```python
from build123d import *

# Parameters (mm, degrees)
F0_W      = 36
F0_H      = 2
F1_DEPTH  = 2
F0_W_2    = 4.0826744884
F0_H_2    = 5.745283328
F2_DEPTH  = 8.5
F3_DEPTH  = 11
F0_W_3    = 2
F4_DEPTH  = 11
F5_W      = 3
F5_H      = 5.745283328
F5_W_2    = 2
F5_W_3    = 1
F6_DEPTH  = 2
F8_DEPTH  = 5.745283328
F10_DEPTH = 5.745283328
F0_W_4    = 3.3082471341
F11_DEPTH = 8


# Not quite as in the source:
# - a feature names something its author has since deleted; it is built from what else it names


with BuildPart() as f1:
    # F0 (on Top) → F1 (new body)
    with BuildSketch(Plane.XY):
        with Locations((0, -10)):
            Rectangle(F0_W, F0_H)
        Polygon((-18, -9), (18, -9), (18, -2.872641664), (14.6917528659, -2.872641664), (14.6917528659, 2.872641664), (18, 2.872641664), (18, 9), (-18, 9), (-18, 2.872641664), (-13.9173255116, 2.872641664), (-13.9173255116, -2.872641664), (-18, -2.872641664), align=None)
    extrude(amount=F1_DEPTH)

    # F0 (on Top) → F2 (join)
    with BuildSketch(Plane.XY):
        with Locations((-15.9586627558, 0)):
            Rectangle(F0_W_2, F0_H_2)
    extrude(amount=F2_DEPTH)

    # F0 (on Top) → F3 (join)
    with BuildSketch(Plane.XY):
        with Locations((0, -10)):
            Rectangle(F0_W, F0_H)
        with Locations((0, 10)):
            Rectangle(F0_W, F0_H)
    extrude(amount=F3_DEPTH)

    # F0 (on Top) → F4 (join)
    with BuildSketch(Plane.XY):
        with Locations((-19, 0)):
            Rectangle(F0_W_3, F0_H_2)
        with Locations((19, 0)):
            Rectangle(F0_W_3, F0_H_2)
    extrude(amount=F4_DEPTH)

    # F5 (on face) → F6 (join)
    with BuildSketch(Plane.XY.offset(11)):
        with Locations((18.5, 0)):
            Rectangle(F5_W, F5_H)
        with Locations((-19, 0)):
            Rectangle(F5_W_2, F5_H)
        with Locations((-17.5, 0)):
            Rectangle(F5_W_3, F5_H)
    extrude(amount=F6_DEPTH)

    # F7 (on face) → F8 (cut, through all)
    with BuildSketch(Plane.XZ.offset(2.872641664)):
        Polygon((-20, 13), (-17, 11), (-17, 13), align=None)
    extrude(amount=-F8_DEPTH, mode=Mode.SUBTRACT)

    # F9 (on face) → F10 (cut, through all)
    with BuildSketch(Plane.XZ.offset(2.872641664)):
        Polygon((17, 13), (17, 11), (20, 13), align=None)
    extrude(amount=-F10_DEPTH, mode=Mode.SUBTRACT)

    # F0 (on Top) → F11 (join)
    with BuildSketch(Plane.XY):
        with Locations((16.345876433, 0)):
            Rectangle(F0_W_4, F0_H_2)
    extrude(amount=F11_DEPTH)


solid = f1.part
```
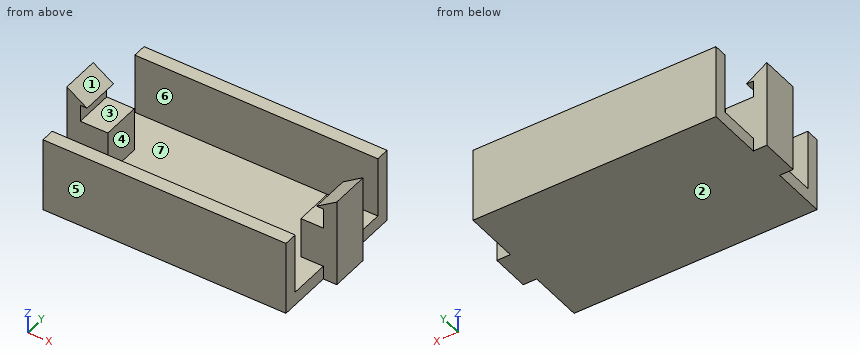
Design review of the part built by this model. Coordinates are the model's own, in mm. Face numbers are marked on the shaded views. A direction names the side the tool comes from. Give positions to 0.01 mm unless a question says otherwise; leave off trailing zeros. Loops run counter-clockwise (first coordinate to the right, second up) from the corner with the lowest first, then second, coordinate; pieces in that order, holes last. Notation, with made-up numbers: M 46.25,6 L 82.25,6 A29 cw 82.25,28 Z; hole C 8.25,9 d6. An arc over 180 degrees is marked long. Return JSON: item names as keys, results as strings. Group by question number.
Item 1: Tool access review of the marked faces 5, 6 and 7: name each direction out of +Z, -Z, +X, -X, +Y, -Y from which nothing blocks a thin tool from reaching the whole face with its end or side.
Item 2: Mouldability with a two-part tool opening along Z and no side actions: class the marked faces 1, 2, 3 and 4 as released by +Z, released by -Z, zero draft, split by the parting line, or undercut.
Item 3: Insertion check: pin 1 Ø3.5 at (x, y) = (-16, -0.5) entering from +Z; pin 2 Ø6.5 at (y, z) = (7, 7) entering from -X; pin 3 Ø1 at (x, y) = (15.5, -1) entering from +Z. Each pin has a flat end and moves straight along its axis. Give the tip position at first contact, or say it passes through.
Item 4: For probe 1 along Y at (x, z) = (-16.5, 4); probe 2 along X at (y, z) = (2.5, 6); probe 3 along Y at (x, z) = (-9.5, 9), list the stretches that pass through material, from the lowest coordinate up.
Item 5: We need section A-A (z = 4.75). Give the boundary of the cut face in (x, y).
Item 6: We need section D-D (z = 1.25). Give the boundary of the cut face in (x, y).
Item 7: We need section C-C (x = 5). Give the boundary of the cut face in (y, z), and give its area (3 significant figures).
Item 8: We need section B-B (y = 1.5). Give the boundary of the cut face in (x, z).
Output:
{
 "1": {"face 5": "+Z, -Z, +X, -X, -Y", "face 6": "+Z, +X, -X", "face 7": "+Z"},
 "2": {"face 1": "released by +Z", "face 2": "released by -Z", "face 3": "undercut", "face 4": "zero draft"},
 "3": {"pin 1": "stops at z = 11.5", "pin 2": "stops at x = -18", "pin 3": "stops at z = 8"},
 "4": {"probe 1": "y = -11 to -9, -2.87 to 2.87, 9 to 11", "probe 2": "x = -20 to -13.92, 14.69 to 20", "probe 3": "y = -11 to -9, 9 to 11"},
 "5": {"outline": "M -20,-2.87 L -13.92,-2.87 L -13.92,2.87 L -20,2.87 Z; M -18,-11 L 18,-11 L 18,-9 L -18,-9 Z; M -18,9 L 18,9 L 18,11 L -18,11 Z; M 14.69,-2.87 L 20,-2.87 L 20,2.87 L 14.69,2.87 Z"},
 "6": {"outline": "M -20,-2.87 L -18,-2.87 L -18,-11 L 18,-11 L 18,-2.87 L 20,-2.87 L 20,2.87 L 18,2.87 L 18,11 L -18,11 L -18,2.87 L -20,2.87 Z"},
 "7": {"outline": "M -11,0 L 11,0 L 11,11 L 9,11 L 9,2 L -9,2 L -9,11 L -11,11 Z", "area": "80.0 mm^2"},
 "8": {"outline": "M -20,0 L 20,0 L 20,13 L 17,11 L 18,11 L 18,8 L 14.69,8 L 14.69,2 L -13.92,2 L -13.92,8.5 L -18,8.5 L -18,11 L -17,11 L -20,13 Z"}
}
